Geometry check sheet. Reference: drawing and pictorial views, mm from the part's lowest x, y, z. A direction names the side the tool comes from. Coordinates: 2 decimals unless noted, no trailing zeros. Loops run counter-clockwise (first coordinate to the right, second up) from the corner with the lowest first, then second, coordinate; pieces in that order, holes last. Notation, with made-up numbers: (-22, -7) - (-5, -7) arc R6 cw to (-5, 0) - close; hole circle Ø8 at (44.25, 73). An arc over 180 degrees is marked (long way). Use a Markdown table: item, result. Add a question column.
1) Go/stop test with flat-tipped pins: P1, Ø17, axis at y = 22.5, z = 15, coming from the +X side; P2, Ø3.5, axis at x = 2.5, z = 8.5, coming from the +Y side. Record where each tip stops, or that it passes through.
2) Tool access check on the marked faces 4, 5 and 6. Record the directions out of +Z, -Z, +X, -X, +Y, -Y that give a thin tool (end or side, any length) a straight path to the whole face; none if there is none.
3) Sectioned sample at B-B, the plane y = 22.5. Enter the section's corners in (x, z).
4) Thickness scan on line 1 (Y direction, x = 23.05, z = 15); line 2 (X direction, y = 17, z = 6); line 3 (X direction, y = 6.5, z = 4.5). Record the ranges inside material, lowest first.
5) Draft check along Y on the marked faces 1, 2 and 3. Enter one of: pulls with the +Y half, pulls with the -Y half, needs draft (parallel to the pull), parting line crosses it, or undercut.
6) Sectioned sample at D-D, the plane z = 4. Enter the section's corners in (x, y).
7) Sectioned sample at A-A, the plane z = 15. Enter the section's corners in (x, y).
8) Sectioned sample at C-C, the plane x = 10. Enter the section's corners in (y, z) (1 decimal).
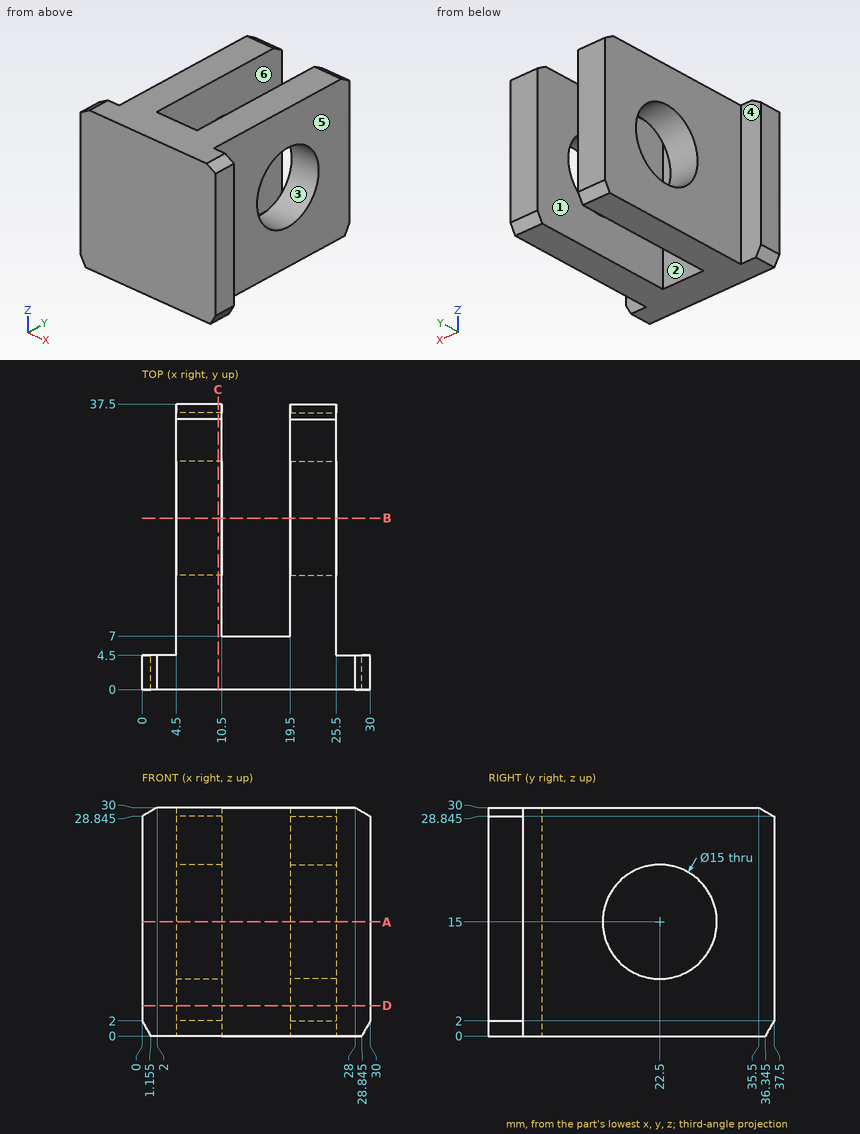
Solved:
| question | item | result |
|---|---|---|
| 1 | P1 | stops at x = 25.5 |
| 1 | P2 | stops at y = 4.5 |
| 2 | face 4 | +Z, -Z, -X, +Y |
| 2 | face 5 | +Z, -Z, +X, +Y |
| 2 | face 6 | +Z, -Z, +Y |
| 3 | outline | (4.5, 0) - (10.5, 0) - (10.5, 7.5) - (4.5, 7.5) - close; (4.5, 22.5) - (10.5, 22.5) - (10.5, 30) - (4.5, 30) - close; (19.5, 0) - (25.5, 0) - (25.5, 7.5) - (19.5, 7.5) - close; (19.5, 22.5) - (25.5, 22.5) - (25.5, 30) - (19.5, 30) - close |
| 4 | line 1 | y = 0 to 15, 30 to 37.5 |
| 4 | line 2 | x = 4.5 to 10.5, 19.5 to 25.5 |
| 4 | line 3 | x = 4.5 to 25.5 |
| 5 | face 1 | needs draft |
| 5 | face 2 | pulls with the +Y half |
| 5 | face 3 | undercut |
| 6 | outline | (0, 0) - (30, 0) - (30, 4.5) - (25.5, 4.5) - (25.5, 37.5) - (19.5, 37.5) - (19.5, 7) - (10.5, 7) - (10.5, 37.5) - (4.5, 37.5) - (4.5, 4.5) - (0, 4.5) - close |
| 7 | outline | (0, 0) - (30, 0) - (30, 4.5) - (25.5, 4.5) - (25.5, 15) - (19.5, 15) - (19.5, 7) - (10.5, 7) - (10.5, 15) - (4.5, 15) - (4.5, 4.5) - (0, 4.5) - close; (4.5, 30) - (10.5, 30) - (10.5, 37.5) - (4.5, 37.5) - close; (19.5, 30) - (25.5, 30) - (25.5, 37.5) - (19.5, 37.5) - close |
| 8 | outline | (0, 0) - (36.3, 0) - (37.5, 2) - (37.5, 28.8) - (35.5, 30) - (0, 30) - close; hole circle Ø15 at (22.5, 15) |
